from build123d import *

# Parameters (mm, degrees)
SKETCH1_W             = 60
SKETCH1_H             = 68
BOSS_EXTRUDE1_DEPTH   = 1.7
SKETCH2_W             = 10
SKETCH2_H             = 29
BOSS_EXTRUDE2_DEPTH   = 22
SKETCH3_W             = 19.649144156
SKETCH3_H             = 20.516018163
BOSS_EXTRUDE3_DEPTH   = 18
SKETCH4_W             = 15
SKETCH4_H             = 13.5
BOSS_EXTRUDE4_DEPTH   = 15
SKETCH5_W             = 13.544906357
SKETCH5_H             = 5.539926829
SKETCH5_H_2           = 5.827547791
CUT_EXTRUDE2_DEPTH    = 13
SKETCH6_W             = 9.824572078
SKETCH6_H             = 11.499215045
BOSS_EXTRUDE5_DEPTH   = 4
SKETCH6_W_2           = 9.098893459
SKETCH6_H_2           = 10.941000723
BOSS_EXTRUDE5_2_DEPTH = 4
SKETCH7_W             = 1.787089801
SKETCH7_H             = 6.912356929
SKETCH7_W_2           = 1.768225957
SKETCH7_W_3           = 1.507178671
SKETCH7_W_4           = 1.674642967
SKETCH7_H_2           = 6.465785471
SKETCH7_W_5           = 1.909421345
SKETCH7_W_6           = 1.332290294
BOSS_EXTRUDE6_DEPTH   = 1
SKETCH8_W             = 10.656311419
SKETCH8_H             = 16.762617894
SKETCH8_W_2           = 9.189366045
SKETCH8_H_2           = 15.720989968
BOSS_EXTRUDE7_DEPTH   = 1
SKETCH9_W             = 1.321363234
SKETCH9_H             = 1.321363233
SKETCH9_W_2           = 1.321363233
SKETCH9_H_2           = 1.321363234
SKETCH9_W_3           = 1.517029512
SKETCH9_H_3           = 1.30031101
SKETCH9_H_4           = 1.269763662
SKETCH9_H_5           = 1.300311011
SKETCH9_W_4           = 1.517029513
BOSS_EXTRUDE8_DEPTH   = 12
SKETCH10_W            = 8.373214839
SKETCH10_H            = 10.941000724
SKETCH10_W_2          = 8.763964865
SKETCH10_H_2          = 10.550250698
SKETCH10_W_3          = 8.652322001
SKETCH10_W_4          = 8.596500568
SKETCH10_H_3          = 10.159500672
BOSS_EXTRUDE9_DEPTH   = 4
SKETCH11_W            = 8.819786297
SKETCH11_H            = 12.113250801
SKETCH11_W_2          = 9.545464917
SKETCH11_H_2          = 12.615643692
SKETCH11_W_3          = 10.129411828
SKETCH11_W_4          = 9.423101323
SKETCH11_H_3          = 11.858861387
BOSS_EXTRUDE10_DEPTH  = 1


with BuildPart() as part:
    # Sketch1 → Boss-Extrude1 (new body)
    with BuildSketch(Plane(origin=(0, 0, 0), x_dir=(1, 0, 0), z_dir=(0, 1, 0))):
        with Locations((-2.434210526, -20.447368421)):
            Rectangle(SKETCH1_W, SKETCH1_H)
    extrude(amount=BOSS_EXTRUDE1_DEPTH)

    # Sketch2 → Boss-Extrude2 (add)
    with BuildSketch(Plane(origin=(0, 1.7, 0), x_dir=(1, 0, 0), z_dir=(0, 1, 0))):
        with Locations((1.565789474, -11.947368421)):
            Rectangle(SKETCH2_W, SKETCH2_H)
    extrude(amount=BOSS_EXTRUDE2_DEPTH)

    # Sketch3 → Boss-Extrude3 (add)
    with BuildSketch(Plane(origin=(0, 1.7, 0), x_dir=(1, 0, 0), z_dir=(0, 1, 0))):
        with Locations((1.358363254, -12.356544357)):
            Rectangle(SKETCH3_W, SKETCH3_H)
    extrude(amount=BOSS_EXTRUDE3_DEPTH)

    # Sketch4 → Boss-Extrude4 (add)
    with BuildSketch(Plane(origin=(0, 1.7, 0), x_dir=(1, 0, 0), z_dir=(0, 1, 0))):
        with Locations((-20.934210526, -47.697368421)):
            Rectangle(SKETCH4_W, SKETCH4_H)
    extrude(amount=BOSS_EXTRUDE4_DEPTH)

    # Sketch5 → Cut-Extrude2 (cut)
    with BuildSketch(Plane.XY.offset(54.447368421)):
        with Locations((-20.953791583, 12.977597446)):
            Rectangle(SKETCH5_W, SKETCH5_H)
        with Locations((-20.953791583, 5.306966548)):
            Rectangle(SKETCH5_W, SKETCH5_H_2)
    extrude(amount=-CUT_EXTRUDE2_DEPTH, mode=Mode.SUBTRACT)



with BuildPart() as body_2:
    # Sketch6 → Boss-Extrude5 (new body)
    with BuildSketch(Plane(origin=(27.565789474, 0, 0), x_dir=(0, 0, -1), z_dir=(1, 0, 0))):
        with Locations((-23.322172183, 12.798964349)):
            Rectangle(SKETCH6_W, SKETCH6_H)
    extrude(amount=-BOSS_EXTRUDE5_DEPTH)


with BuildPart() as body_3:
    # Sketch6 → Boss-Extrude5 2 (new body)
    with BuildSketch(Plane(origin=(27.565789474, 0, 0), x_dir=(0, 0, -1), z_dir=(1, 0, 0))):
        with Locations((-3.645117311, 12.519857188)):
            Rectangle(SKETCH6_W_2, SKETCH6_H_2)
    extrude(amount=-BOSS_EXTRUDE5_2_DEPTH)


with BuildPart() as part_1:
    add(part.part)

    add(body_2.part)  # Boss-Extrude6 merges body 2

    add(body_3.part)  # Boss-Extrude6 merges body 3
    # Sketch7 → Boss-Extrude6 (add)
    with BuildSketch(Plane(origin=(27.565789474, 0, 0), x_dir=(0, 0, -1), z_dir=(1, 0, 0))):
        with Locations((-27.340913322, 5.156178464)):
            Rectangle(SKETCH7_W, SKETCH7_H)
        with Locations((-23.498666417, 5.156178464)):
            Rectangle(SKETCH7_W_2, SKETCH7_H)
        with Locations((-20.056618396, 5.156178464)):
            Rectangle(SKETCH7_W_3, SKETCH7_H)
        with Locations((-6.46409964, 4.932892736)):
            Rectangle(SKETCH7_W_4, SKETCH7_H_2)
        with Locations((-3.053245947, 4.932892736)):
            Rectangle(SKETCH7_W_5, SKETCH7_H_2)
        with Locations((-0.439096995, 4.932892736)):
            Rectangle(SKETCH7_W_6, SKETCH7_H_2)
    extrude(amount=-BOSS_EXTRUDE6_DEPTH)

    # Sketch8 → Boss-Extrude7 (add)
    with BuildSketch(Plane(origin=(27.565789474, 0, 0), x_dir=(0, 0, -1), z_dir=(1, 0, 0))):
        with Locations((-23.292544957, 14.912084667)):
            Rectangle(SKETCH8_W, SKETCH8_H)
        with Locations((-3.65570245, 14.483934281)):
            Rectangle(SKETCH8_W_2, SKETCH8_H_2)
    extrude(amount=-BOSS_EXTRUDE7_DEPTH)

    # Sketch9 → Boss-Extrude8 (add)
    with BuildSketch(Plane(origin=(0, 1.7, 0), x_dir=(1, 0, 0), z_dir=(0, 1, 0))):
        with Locations((-29.367713838, -1.42279795)):
            Rectangle(SKETCH9_W, SKETCH9_H)
        with Locations((-29.670931722, 11.160296109)):
            Rectangle(SKETCH9_W_2, SKETCH9_H_2)
        with Locations((-29.639547043, 8.60572197)):
            Rectangle(SKETCH9_W_3, SKETCH9_H_3)
        with Locations((-29.639547043, 5.989826275)):
            Rectangle(SKETCH9_W_3, SKETCH9_H_4)
        with Locations((-29.336329159, -3.97737209)):
            Rectangle(SKETCH9_W_3, SKETCH9_H_5)
        with Locations((-29.336329159, -6.593267784)):
            Rectangle(SKETCH9_W_3, SKETCH9_H_4)
        with Locations((-29.357446593, -14.692498665)):
            Rectangle(SKETCH9_W_2, SKETCH9_H)
        with Locations((-29.326061914, -17.247072804)):
            Rectangle(SKETCH9_W_3, SKETCH9_H_3)
        with Locations((-29.326061914, -19.862968498)):
            Rectangle(SKETCH9_W_3, SKETCH9_H_4)
        with Locations((-29.34335534, -26.079899051)):
            Rectangle(SKETCH9_W, SKETCH9_H)
        with Locations((-29.311970662, -28.63447319)):
            Rectangle(SKETCH9_W_4, SKETCH9_H_3)
        with Locations((-29.311970662, -31.250368885)):
            Rectangle(SKETCH9_W_4, SKETCH9_H_4)
    extrude(amount=BOSS_EXTRUDE8_DEPTH)

    # Sketch10 → Boss-Extrude9 (add)
    with BuildSketch(Plane.ZY.offset(30.331613338)):
        with Locations((-8.496044207, 11.235964245)):
            Rectangle(SKETCH10_W, SKETCH10_H)
        with Locations((3.86840304, 11.040589232)):
            Rectangle(SKETCH10_W_2, SKETCH10_H_2)
        with Locations((17.823761105, 11.040589232)):
            Rectangle(SKETCH10_W_3, SKETCH10_H_2)
        with Locations((28.792672544, 10.845214219)):
            Rectangle(SKETCH10_W_4, SKETCH10_H_3)
    extrude(amount=-BOSS_EXTRUDE9_DEPTH)

    # Sketch11 → Boss-Extrude10 (add)
    with BuildSketch(Plane.ZY.offset(30.331613338)):
        with Locations((-8.32857991, 13.385089388)):
            Rectangle(SKETCH11_W, SKETCH11_H)
        with Locations((4.147510201, 13.133892942)):
            Rectangle(SKETCH11_W_2, SKETCH11_H_2)
        with Locations((17.836627399, 13.385089388)):
            Rectangle(SKETCH11_W_3, SKETCH11_H)
        with Locations((28.841568651, 13.512284095)):
            Rectangle(SKETCH11_W_4, SKETCH11_H_3)
    extrude(amount=-BOSS_EXTRUDE10_DEPTH)


solid = part_1.part
Here's how the part is built. I have some questions about the finished solid (model axes, mm). A direction names the side the tool comes from. Give positions to 0.01 mm unless a question says otherwise; leave off trailing zeros. Order: outer loops, then holes, each group sorted by start corner. A loop starts at its lowest first (then second) coordinate and runs counter-clockwise, first axis right, second up. Notation, with made-up numbers: M 48.25,37.5 L 71.25,37.5 A14 ccw 71.25,49.5 Z; hole C 37,13.25 d3. An arc over 180 degrees is marked long. Answer as a JSON object with one key per item and string values. Group by question number.
1) Suppose I cut it at A-A, the plane z = 48. Write out the boundary of the cut face in (x, y).
2) On a 3-axis mill with a long thin cutter (end or side, diameter ignored), from which of +Z, -Z, +X, -X, +Y, -Y can I reach the whole of each face in a straight line? I mean faces 4 (the flat face through (-6, 11, 2.099)), 5 (the flat face through (-28, 16.316, 4)), 6 (the flat face through (-26.332, 11, -9)), 7 (the flat face through (-14.181, 5, 48)), 8 (the flat face through (25, 18.549, 23)). Say none if no direction works.
3) Suppose I cut it at B-B, the plane x = -23. Write out the boundary of the cut face in (y, z), plus the area to 3 significant figures.
4) Please list where these lines run through material, in increasing order: L1, parallel to X at y = 16.75, z = 6; L2, parallel to X at y = 3.25, z = 6; L3, parallel to Z at x = -26.5, y = 10.5. Write a range as [from, to].
5) Suppose I cut it at C-C, the plane x = -4.5. Write out the boundary of the cut face in (y, z).
6) We'd pull the mould along X, two halves only. Please class faces 1 (the flat face through (1, 13, 26.447)), 2 (the flat face through (-28, 5.765, -9)), 3 (the flat face through (-30.332, 13, 4)): pulls with the +X half, pulls with the -X half, needs draft (parallel to the pull), parting line crosses it, or undercut.
7) Suppose I cut it at D-D, the plane x = 5. Write out the boundary of the cut face in (y, z).
8) I'm going to push flat-ended pins straight in: pin 1 Ø3 at (y, z) = (5, 44.5) entering from -X; pin 2 Ø4 at (x, y) = (10.5, 20) entering from -Z; pin 3 Ø0.8 at (x, y) = (-29, 3.5) entering from -Z; pin 4 Ø2 at (y, z) = (4.5, 38) entering from -X. Where does each tip first touch, or does it pass through?
Results found:
{
 "1": {"outline": "M -32.43,0 L 27.57,0 L 27.57,1.7 L -13.43,1.7 L -13.43,16.7 L -28.43,16.7 L -28.43,1.7 L -32.43,1.7 Z; hole M -27.73,2.39 L -14.18,2.39 L -14.18,8.22 L -27.73,8.22 Z; hole M -27.73,10.21 L -14.18,10.21 L -14.18,15.75 L -27.73,15.75 Z"},
 "2": {"face 4": "-Z, +Y", "face 5": "+Y", "face 6": "-Z, +X, +Y", "face 7": "+Z", "face 8": "+Z, -Z, +Y"},
 "3": {"outline": "M 0,-13.55 L 1.7,-13.55 L 1.7,40.95 L 16.7,40.95 L 16.7,54.45 L 15.75,54.45 L 15.75,41.45 L 10.21,41.45 L 10.21,54.45 L 8.22,54.45 L 8.22,41.45 L 2.39,41.45 L 2.39,54.45 L 0,54.45 Z", "area": "170 mm²"},
 "4": {"L1": "[-30.33, -29.33], [-8.47, 11.18], [23.57, 27.57]", "L2": "[-30.09, -28.58], [-8.47, 11.18], [26.57, 27.57]", "L3": "[-12.68, -4.31], [-0.51, 8.25], [13.5, 22.15], [24.49, 33.09], [40.95, 41.45]"},
 "5": {"outline": "M 0,-13.55 L 1.7,-13.55 L 1.7,2.1 L 19.7,2.1 L 19.7,22.61 L 1.7,22.61 L 1.7,54.45 L 0,54.45 Z"},
 "6": {"face 1": "undercut", "face 2": "needs draft", "face 3": "pulls with the -X half"},
 "7": {"outline": "M 0,-13.55 L 1.7,-13.55 L 1.7,-2.55 L 23.7,-2.55 L 23.7,26.45 L 1.7,26.45 L 1.7,54.45 L 0,54.45 Z"},
 "8": {"pin 1": "x = -28.43", "pin 2": "z = 2.1", "pin 3": "z = -11.82", "pin 4": "through"}
}
